```python
from build123d import *

# Parameters (mm, degrees)
EXTRUDE_1_DEPTH     = 40
HOLE_WIZARD_M12_1_D = 10.2


with BuildPart() as part:
    # 草图1 → 凸台-拉伸1 (new, symmetric)
    with BuildSketch(Plane.XY):
        Polygon((0, 0), (0, 47.406641223), (32, 25), (32, 0), align=None)
    extrude(amount=EXTRUDE_1_DEPTH, both=True)

    # M12 螺纹孔1 (through all)
    with Locations(Plane(origin=(32, 0, 0), x_dir=(0, 0, -1), z_dir=(1, 0, 0))):
        with Locations((-25, 11), (25, 11)):
            Hole(HOLE_WIZARD_M12_1_D / 2)


solid = part.part
```
Geometry check sheet. Reference: the model listing, model coordinates, mm. Coordinates: 2 decimals unless noted, no trailing zeros. Order: outer loops, then holes, each group sorted by start corner. A loop starts at its lowest first (then second) coordinate and runs counter-clockwise, first axis right, second up. Notation, with made-up numbers: M 8.5,15 L 45.5,15 A25 cw 45.5,49 Z; hole C -32.5,36.25 d5. An arc over 180 degrees is marked long. One line per question, with ' | ' between items. Start each with the question number.
Item 1: Cross-section at C-C on x = 7. Enter the section's corners in (y, z), then the cut area to 3 significant figures.
Item 2: Cross-section at D-D on z = 27.5. Enter the section's corners in (x, y).
Item 3: Material ranges on L1, parallel to Y at x = 22, z = -25; L2, parallel to Y at x = 10, z = 25; L3, parallel to X at y = 43.5, z = 7, recorded low to high. Write a range as [from, to].
Item 4: Cross-section at A-A on y = 11. Enter the section's corners in (x, z), then the cut area to 3 significant figures.
Item 5: Cross-section at B-B on z = -25. Enter the section's corners in (x, y), then the cut area to 3 significant figures.
Item 6: Draft check along Y on faces 1 (the flat face through (16, 0, 1)), 2 (the cylindrical face through (15.776, 11.224, 19.905)), 3 (the flat face through (16, 19, 40)), 4 (the flat face through (15.776, 36.36, 0.56)). Enter one of: pulls with the +Y half, pulls with the -Y half, needs draft (parallel to the pull), parting line crosses it, or undercut.
Item 7: Gauge pin test, flat ends, axial feed: pin 1 (3 mm diameter, centred on y = 29, z = 13, fed in from -X); pin 2 (12 mm diameter, centred on x = 22, z = 26.5, fed in from +Y). Record the tip position at first contact, or that the pin passes through.
Findings:
1) outline: M 0,-40 L 42.51,-40 L 42.51,40 L 0,40 Z; hole C 11,-25 d10.2; hole C 11,25 d10.2 | area: 3,240 mm²
2) outline: M 0,0 L 32,0 L 32,6.55 L 0,6.55 Z; M 0,15.45 L 32,15.45 L 32,25 L 0,47.41 Z
3) L1: y = [0, 5.9], [16.1, 32] | L2: y = [0, 5.9], [16.1, 40.4] | L3: x = [0, 5.58]
4) outline: M 0,-40 L 32,-40 L 32,-30.1 L 0,-30.1 Z; M 0,-19.9 L 32,-19.9 L 32,19.9 L 0,19.9 Z; M 0,30.1 L 32,30.1 L 32,40 L 0,40 Z | area: 1,910 mm²
5) outline: M 0,0 L 32,0 L 32,5.9 L 0,5.9 Z; M 0,16.1 L 32,16.1 L 32,25 L 0,47.41 Z | area: 832 mm²
6) face 1: pulls with the -Y half | face 2: undercut | face 3: needs draft | face 4: pulls with the +Y half
7) pin 1: stops at x = 0 | pin 2: stops at y = 36.2
